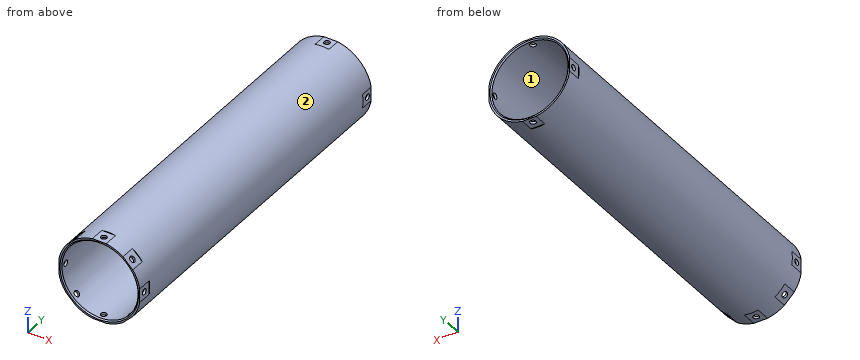
```python
from build123d import *

# Parameters (mm, degrees)
F_1_4_0_25_DIAMETER_HOLE1_REACH  = 395.014
F_1_4_0_25_DIAMETER_HOLE1_BORE_R = 3.175
CIRPATTERN2_COUNT                = 4
CHAMFER1_SIZE                    = 1.27
CIRPATTERN1_COUNT                = 8
SKETCH7_W                        = 16.51
SKETCH7_H                        = 16.51
CUT_EXTRUDE1_DEPTH               = 0.635
SKETCH8_W                        = 16.51
SKETCH8_H                        = 16.51
CUT_EXTRUDE2_DEPTH               = 0.635
CIRPATTERN4_COUNT                = 8
CIRPATTERN5_COUNT                = 4


with BuildPart() as part:
    # Sketch2 → Revolve1 (revolve)
    with BuildSketch(Plane.XY, mode=Mode.PRIVATE) as revolve1_sk:
        Polygon((41.275, 0), (44.45, 0), (44.45, 387.858), (41.275, 387.858), (41.275, 193.929), align=None)
    revolve(revolve1_sk.sketch.rotate(Axis((0, 0, 0), (0, 1, 0)), 90), axis=Axis((0, 0, 0), (0, 1, 0)))

    # 1/4 (0.25) Diameter Hole1 bore (on position points) → 1/4 (0.25) Diameter Hole1 (cut, up to next)
    with BuildSketch(Plane(origin=(0, 7.62, -44.45), x_dir=(-1, 0, 0), z_dir=(0, 0, -1)), mode=Mode.PRIVATE) as f_1_4_0_25_diameter_hole1_sk1:
        Circle(F_1_4_0_25_DIAMETER_HOLE1_BORE_R)
    f_1_4_0_25_diameter_hole1_tool1 = extrude(f_1_4_0_25_diameter_hole1_sk1.sketch, amount=-F_1_4_0_25_DIAMETER_HOLE1_REACH, mode=Mode.PRIVATE) & part.part
    f_1_4_0_25_diameter_hole1 = f_1_4_0_25_diameter_hole1_tool1.solids().sort_by_distance((0, 7.62, -44.45))[0]
    add(f_1_4_0_25_diameter_hole1, mode=Mode.SUBTRACT)

    # Sketch6 → 1/4 (0.25) Diameter Hole2 (revolve, cut)
    with BuildSketch(Plane(origin=(0, 381.508, -44.45), x_dir=(0, 1, 0), z_dir=(1, 0, 0))):
        Polygon((0, 0), (0, 5.209732465), (3.175, 3.302), (3.175, 0), align=None)
    f_1_4_0_25_diameter_hole2 = revolve(axis=Axis((0, 381.508, -50.8), (0, 0, 1)), mode=Mode.SUBTRACT)

    # CirPattern2: 1/4 (0.25) Diameter Hole2 ×4 about axis
    cirpattern2_axis = Axis((0, -17.04721, 0), (0, 1, 0))
    for i in range(1, CIRPATTERN2_COUNT):
        add(f_1_4_0_25_diameter_hole2.rotate(cirpattern2_axis, i * 360 / CIRPATTERN2_COUNT), mode=Mode.SUBTRACT)

    # Chamfer1
    chamfer1_edges = [part.edges().sort_by_distance(p)[0] for p in [
        (0, 387.858, 41.275),
        (0, 0, 41.275),
    ]]
    chamfer(chamfer1_edges, length=CHAMFER1_SIZE)

    # CirPattern1: 1/4 (0.25) Diameter Hole1 ×8 about axis
    cirpattern1_axis = Axis((0, -17.04721, 0), (0, 1, 0))
    for i in range(1, CIRPATTERN1_COUNT):
        add(f_1_4_0_25_diameter_hole1.rotate(cirpattern1_axis, i * 360 / CIRPATTERN1_COUNT), mode=Mode.SUBTRACT)

    # Sketch7 → Cut-Extrude1 (cut)
    with BuildSketch(Plane(origin=(44.45, 0, 0), x_dir=(0, 0, -1), z_dir=(1, 0, 0))):
        with Locations((0, 7.62)):
            Rectangle(SKETCH7_W, SKETCH7_H)
    cut_extrude1 = extrude(amount=-CUT_EXTRUDE1_DEPTH, mode=Mode.SUBTRACT)

    # Sketch8 → Cut-Extrude2 (cut)
    with BuildSketch(Plane(origin=(44.45, 0, 0), x_dir=(0, 0, -1), z_dir=(1, 0, 0))):
        with Locations((0, 381.508)):
            Rectangle(SKETCH8_W, SKETCH8_H)
    cut_extrude2 = extrude(amount=-CUT_EXTRUDE2_DEPTH, mode=Mode.SUBTRACT)

    # CirPattern4: Cut-Extrude1 ×8 about axis
    cirpattern4_axis = Axis((0, 0, 0), (0, 1, 0))
    for i in range(1, CIRPATTERN4_COUNT):
        add(cut_extrude1.rotate(cirpattern4_axis, i * 360 / CIRPATTERN4_COUNT), mode=Mode.SUBTRACT)

    # CirPattern5: Cut-Extrude2 ×4 about axis
    cirpattern5_axis = Axis((0, 0, 0), (0, 1, 0))
    for i in range(1, CIRPATTERN5_COUNT):
        add(cut_extrude2.rotate(cirpattern5_axis, i * 360 / CIRPATTERN5_COUNT), mode=Mode.SUBTRACT)


solid = part.part
```
Geometry check sheet. Reference: the model listing, model coordinates, mm. Face numbers are marked on the shaded views. Coordinates: 2 decimals unless noted, no trailing zeros. Loops run counter-clockwise (first coordinate to the right, second up) from the corner with the lowest first, then second, coordinate; pieces in that order, holes last.
Item 1: Thickness scan on line 1 (Y direction, x = -43.1, z = 0) (3 decimals); line 2 (Z direction, x = -0.5, y = 349); line 3 (Y direction, x = -42.35, z = 0) (3 decimals). Record the ranges inside material, lowest first.
Item 2: Go/stop test with flat-tipped pins: pin 1 Ø11.5 at (x, z) = (-31, -29.5) entering from -Y; pin 2 Ø0.5 at (x, z) = (44.5, 3.5) entering from +Y; pin 3 Ø10 at (y, z) = (243, -9.5) entering from -X; pin 4 Ø3 at (y, z) = (282.5, -20.5) entering from -X. Record where each tip stops, or that it passes through.
Item 3: Release check for a two-part mould opening along Z. For the marked faces 1 and 2 record: released by +Z, released by -Z, zero draft, split by the parting line, or undercut.
Item 4: Sectioned sample at A-A, the plane y = 96.5. Record the boundary of the cut face in (x, z) (3 decimals).
Check result:
1. line 1: y = 0 to 4.445, 10.795 to 378.333, 384.683 to 387.858
1. line 2: z = -44.45 to -41.27, 41.27 to 44.45
1. line 3: y = 0.195 to 4.445, 10.795 to 378.333, 384.683 to 387.663
2. pin 1: stops at y = 0
2. pin 2: stops at y = 373.25
2. pin 3: stops at x = -44.22
2. pin 4: stops at x = -40.18
3. face 1: undercut
3. face 2: split by the parting line
4. outline: circle Ø88.9 at (0, 0); hole circle Ø82.55 at (0, 0)
